Geometry: final body of the model. Coordinates: model frame, mm. Face numbers are marked on the shaded views. A direction names the side the tool comes from. Round coordinates to 2 decimals unless told otherwise and drop trailing zeros. Write each loop counter-clockwise with the first axis right and the second up, starting at its lowest first coordinate (ties: lowest second). Pieces come first, ordered by that corner, then holes. Notation, with made-up numbers: (6, 70.5) -> (26, 70.5) arc R31 cw to (26, 101.5) -> close; hole circle Ø4 at (-15.5, -39.5). An arc over 180 degrees is marked (long way). Use one line per item in the form item = value. Start each with the question number.
1. Cut plane A-A, the plane z = 0. Return the cut outline in (x, y).
2. Cut plane B-B, the plane x = -10. Return the cut outline in (y, z), plus the area to 3 significant figures.
3. Draft query along Z for the marked faces 1, 2, 3 and 4. Return one class per face: pulls with the +Z half, pulls with the -Z half, needs draft (parallel to the pull), parting line crosses it, or undercut.
4. Line query: L1, parallel to X at y = 16.75, z = 0; L2, parallel to Z at x = 4.5, y = 12.5; L3, parallel to Z at x = 35, y = 16. Output: solid intervals per line, ascending.
5. Pin query (flat end, axial travel): pin 1 Ø2.5 at (x, z) = (-15.5, 0) entering from +Y; pin 2 Ø2 at (y, z) = (8.5, -13) entering from +X; pin 3 Ø3.5 at (y, z) = (6.5, 0.5) entering from -X. Return the tip coordinate at first contact, or that it passes through.
6. Cut plane C-C, the plane x = 12. Return the cut outline in (y, z), plus the area to 3 significant figures.
7. Cut plane D-D, the plane y = 12.25. Return the cut outline in (x, z), plus the area to 3 significant figures.
8. Reachability of the marked faces 5, 6, 7, 8 and 9 from +Z, -Z, +X, -X, +Y, -Y: full face, straight path, thin tool, end or side. Return the list, or none.
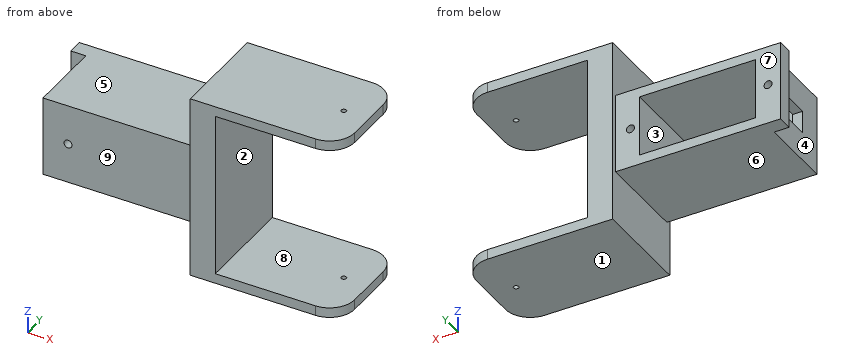
```python
from build123d import *

# Parameters (mm, degrees)
SKETCH1_W               = 30
SKETCH1_H               = 16
BOSS_EXTRUDE1_DEPTH     = 2
SKETCH2_W               = 23.2
SKETCH2_H               = 12.2
BOSS_EXTRUDE2_DEPTH     = 16
CUT_EXTRUDE1_REACH      = 36.234
SKETCH3_W               = 4.5
SKETCH3_H               = 13
SKETCH8_R               = 0.8
CUT_EXTRUDE3_DEPTH      = 2
SKETCH9_W               = 5
SKETCH9_H               = 16
SKETCH9_W_2             = 4
BOSS_EXTRUDE4_DEPTH     = 3
SKETCH10_R              = 0.8
CUT_EXTRUDE4_DEPTH      = 5
SKETCH11_W              = 37
SKETCH11_H              = 20
BOSS_EXTRUDE5_DEPTH     = 5
SKETCH12_W              = 2
SKETCH12_H              = 20
BOSS_EXTRUDE6_DEPTH     = 25
FILLET1_R               = 5
CUT_EXTRUDE5_DEPTH      = 62.278054799
CUT_EXTRUDE5_DEPTH_BACK = 62.278054799
SKETCH13_R              = 0.5


with BuildPart() as part:
    # Sketch1 → Boss-Extrude1 (new body)
    with BuildSketch(Plane(origin=(0, 0, 0), x_dir=(1, 0, 0), z_dir=(0, 1, 0))):
        Rectangle(SKETCH1_W, SKETCH1_H)
    extrude(amount=BOSS_EXTRUDE1_DEPTH)

    # Sketch2 → Boss-Extrude2 (add)
    with BuildSketch(Plane(origin=(0, 2, 0), x_dir=(1, 0, 0), z_dir=(0, 1, 0))):
        Polygon((-15, 8), (-13, 8), (10.2, 8), (15, 8), (15, -8), (10.2, -8), (-13, -8), (-15, -8), align=None)
        with Locations((-1.4, 0)):
            Rectangle(SKETCH2_W, SKETCH2_H, mode=Mode.SUBTRACT)
    extrude(amount=BOSS_EXTRUDE2_DEPTH)

    # Sketch3 → Cut-Extrude1 (cut, up to next)
    with BuildSketch(Plane(origin=(-13, 0, 0), x_dir=(0, 0, -1), z_dir=(1, 0, 0)), mode=Mode.PRIVATE) as cut_extrude1_sk1:
        with Locations((0, 11.5)):
            Rectangle(SKETCH3_W, SKETCH3_H)
    cut_extrude1_tool1 = extrude(cut_extrude1_sk1.sketch, amount=-CUT_EXTRUDE1_REACH, mode=Mode.PRIVATE) & part.part
    add(cut_extrude1_tool1.solids().sort_by_distance((-13, 11.5, 0))[0], mode=Mode.SUBTRACT)

    # Sketch8 → Cut-Extrude3 (cut)
    with BuildSketch(Plane.XZ):
        with Locations(Location((-10, 0, 0), (0, 0, 270))):
            Circle(SKETCH8_R)
    extrude(amount=-CUT_EXTRUDE3_DEPTH, mode=Mode.SUBTRACT)

    # Sketch9 → Boss-Extrude4 (add)
    with BuildSketch(Plane(origin=(0, 18, 0), x_dir=(1, 0, 0), z_dir=(0, 1, 0))):
        with Locations((-15.5, 0)):
            Rectangle(SKETCH9_W, SKETCH9_H)
        with Locations((12.2, 0)):
            Rectangle(SKETCH9_W_2, SKETCH9_H)
    extrude(amount=-BOSS_EXTRUDE4_DEPTH)

    # Sketch10 → Cut-Extrude4 (cut)
    with BuildSketch(Plane(origin=(0, 18, 0), x_dir=(1, 0, 0), z_dir=(0, 1, 0))):
        with Locations(Location((12, 0, 0), (0, 0, 270))):
            Circle(SKETCH10_R)
        with Locations(Location((-15.500971551, 0, 0), (0, 0, 270))):
            Circle(SKETCH10_R)
    extrude(amount=-CUT_EXTRUDE4_DEPTH, mode=Mode.SUBTRACT)

    # Sketch11 → Boss-Extrude5 (add)
    with BuildSketch(Plane(origin=(15, 0, 0), x_dir=(0, 0, -1), z_dir=(1, 0, 0))):
        with Locations((0, 9)):
            Rectangle(SKETCH11_W, SKETCH11_H)
    extrude(amount=BOSS_EXTRUDE5_DEPTH)

    # Sketch12 → Boss-Extrude6 (add)
    with BuildSketch(Plane(origin=(20, 0, 0), x_dir=(0, 0, -1), z_dir=(1, 0, 0))):
        with Locations((-17.5, 9)):
            Rectangle(SKETCH12_W, SKETCH12_H)
        with Locations((17.5, 9)):
            Rectangle(SKETCH12_W, SKETCH12_H)
    extrude(amount=BOSS_EXTRUDE6_DEPTH)

    # Fillet1
    fillet1_edges = [part.edges().sort_by_distance(p)[0] for p in [
        (45, 19, -17.5),
        (45, -1, -17.5),
        (45, 19, 17.5),
        (45, -1, 17.5),
    ]]
    fillet(fillet1_edges, radius=FILLET1_R)

    # Sketch13 → Cut-Extrude5 (cut, two sides: drawn at the far end of the back side and taken through both)
    with BuildSketch(Plane(origin=(0, 0, -18.5), x_dir=(-1, 0, 0), z_dir=(0, 0, -1)).offset(-CUT_EXTRUDE5_DEPTH_BACK)):
        with Locations((-40, 9)):
            Circle(SKETCH13_R)
    extrude(amount=CUT_EXTRUDE5_DEPTH + CUT_EXTRUDE5_DEPTH_BACK, mode=Mode.SUBTRACT)


solid = part.part
```
Outcome:
q1.outline = (-18, 15) -> (-16.3, 15) -> (-16.3, 18) -> (-18, 18) -> close; (-15, 0) -> (-10.8, 0) -> (-10.8, 2) -> (-13, 2) -> (-13, 5) -> (-15, 5) -> close; (-14.7, 15) -> (-13, 15) -> (-13, 18) -> (-14.7, 18) -> close; (-9.2, 0) -> (15, 0) -> (15, -1) -> (20, -1) -> (20, 19) -> (15, 19) -> (15, 18) -> (12.8, 18) -> (12.8, 13) -> (11.2, 13) -> (11.2, 18) -> (10.2, 18) -> (10.2, 2) -> (-9.2, 2) -> close
q2.outline = (0, -8) -> (18, -8) -> (18, -6.1) -> (2, -6.1) -> (2, -0.8) -> (0, -0.8) -> close; (0, 0.8) -> (2, 0.8) -> (2, 6.1) -> (18, 6.1) -> (18, 8) -> (0, 8) -> close
q2.area = 89.6 mm^2
q3.face_1 = pulls with the -Z half
q3.face_2 = undercut
q3.face_3 = undercut
q3.face_4 = needs draft
q4.L1 = -18 to -16.3, -14.7 to -13, 10.2 to 11.2, 12.8 to 20
q4.L2 = -8 to -6.1, 6.1 to 8
q4.L3 = -18.5 to -16.5, 16.5 to 18.5
q5.pin_1 = 18
q5.pin_2 = 20
q5.pin_3 = -15
q6.outline = (0, -8) -> (18, -8) -> (18, -0.8) -> (13, -0.8) -> (13, 0.8) -> (18, 0.8) -> (18, 8) -> (0, 8) -> close
q6.area = 280 mm^2
q7.outline = (-15, -8) -> (15, -8) -> (15, -18.5) -> (45, -18.5) -> (45, -16.5) -> (20, -16.5) -> (20, 16.5) -> (45, 16.5) -> (45, 18.5) -> (15, 18.5) -> (15, 8) -> (-15, 8) -> (-15, 2.25) -> (-13, 2.25) -> (-13, 6.1) -> (10.2, 6.1) -> (10.2, -6.1) -> (-13, -6.1) -> (-13, -2.25) -> (-15, -2.25) -> close
q7.area = 473 mm^2
q8.face_5 = +Z, -X, +Y, -Y
q8.face_6 = -Z, -X, +Y, -Y
q8.face_7 = +Z, -Z, -X, +Y
q8.face_8 = +X, +Y, -Y
q8.face_9 = +Z, -Z, -X, -Y
